Work out the finished part from the listing and answer in its coordinate system (mm). Face numbers are marked on the shaded views. Round coordinates to 2 decimals unless told otherwise and drop trailing zeros. Order: outer loops, then holes, each group sorted by start corner. A loop starts at its lowest first (then second) coordinate and runs counter-clockwise, first axis right, second up. Notation, with made-up numbers: (-32, 8) -> (-4, 8) arc R29 ccw to (-4, 42) -> close; hole circle Ø11 at (-13, -29). An arc over 180 degrees is marked (long way). Use one line per item in the form item = value.
Autodesk Inventor part; units mm, degrees
ref_plane "YZ Plane" through (0, 0, 0) normal (1, 0, 0) x (0, 1, 0)
ref_plane "XZ Plane" through (0, 0, 0) normal (0, 1, 0) x (-1, 0, 0)
ref_plane "XY Plane" through (0, 0, 0) normal (0, 0, 1) x (1, 0, 0)
sketch "Sketch1" plane through (0, 0, 0) normal (0, 1, 0) x (-1, 0, 0)
  circle A0 centre (0, 0) radius 3.2
  circle A1 centre (0, 0) radius 6.5
  line L0 (-2.7713, 1.6) -> (2.7713, 1.6)
  dimension "d0" = 6.4
  dimension "d2" = 13
  dimension "d7" = 4.8
extrude "Extrusion1" add sketch "Sketch1" along normal blind 11 contours A0 L0 | L0 A0 | A1
extrude "Extrusion2" cut sketch "Sketch1" along normal blind 2.7 contours A0 L0 | L0 A0
extrude "Extrusion3" cut sketch "Sketch1" along normal blind 9.7 contours A0 L0 picked at (-0.1715, -0.3975)
sketch "Sketch3" plane through (0, 0, 0) normal (1, 0, 0) x (0, 1, 0)
  line L0 (0, 6.5) -> (11, 6.5)
  line L1 (11, 6.5) -> (11, -6.5)
  line L2 (11, -6.5) -> (0, -6.5)
  line L3 (0, -6.5) -> (0, -3.2)
  line L4 (0, -3.2) -> (9.7, -3.2)
  line L5 (9.7, -3.2) -> (9.7, 1.6)
  line L6 (9.7, 1.6) -> (2.7, 1.6)
  line L7 (2.7, 1.6) -> (2.7, 3.2)
  line L8 (2.7, 3.2) -> (0, 3.2)
  line L9 (0, 3.2) -> (0, 6.5)
  line L10 (11, 1.9375) -> (7, 6.5)
  point P0 (0, 0)
  dimension "d12" = 1.2
  dimension "d13" = 7
extrude "Extrusion5" cut sketch "Sketch3" along normal through all both and the other way through all contours L0 L1 L10
equation "\"offset\" = 0.2"
properties part number "knob"
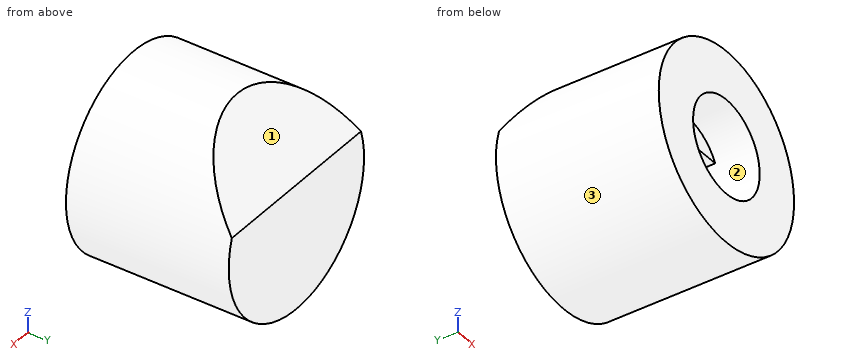
Item 1: The part is cut by section A-A, the plane x = 0. Give the vertices of the cut face in (y, z), and give its area (3 significant figures).
Findings:
outline = (0, -6.5) -> (11, -6.5) -> (11, 1.94) -> (7, 6.5) -> (0, 6.5) -> (0, 3.2) -> (2.7, 3.2) -> (2.7, 1.6) -> (9.7, 1.6) -> (9.7, -3.2) -> (0, -3.2) -> close
area = 83.0 mm^2
Item 2: Consider line 1 along Z through (x, y) = (0, 5.5); line 2 along X through (y, z) = (4.5, 0); line 3 along Z through (x, y) = (-1.5, 3.75). Determine where each line is inside the solid, lowest interval first.
Findings:
line_1 = -6.5 to -3.2, 1.6 to 6.5
line_2 = -6.5 to -3.2, 3.2 to 6.5
line_3 = -6.32 to -2.83, 1.6 to 6.32
Item 3: The part is cut by section D-D, the plane x = 2.5. Give the vertices of the cut face in (y, z), and give its area (3 significant figures).
Findings:
outline = (0, -6) -> (11, -6) -> (11, 1.94) -> (7.44, 6) -> (0, 6) -> (0, 2) -> (2.7, 2) -> (2.7, 1.6) -> (9.7, 1.6) -> (9.7, -2) -> (0, -2) -> close
area = 88.8 mm^2
Item 4: Determine the mould class of the marked faces 1, 2 and 3 for opening direction X: released by +X, released by -X, zero draft, split by the parting line, or undercut.
Findings:
face_1 = zero draft
face_2 = undercut
face_3 = split by the parting line
Item 5: The part is cut by section C-C, the plane z = -0.5. Give the vertices of the cut face in (x, y), and give its area (3 significant figures).
Findings:
outline = (-6.48, 0) -> (-3.16, 0) -> (-3.16, 9.7) -> (3.16, 9.7) -> (3.16, 0) -> (6.48, 0) -> (6.48, 11) -> (-6.48, 11) -> close
area = 81.3 mm^2
Item 6: Flat-ended cylindrical pins translate along their axes: P1, Ø2, axis at x = 3.5, y = 2, coming from the +Z side; P2, Ø1.3, axis at x = 1, z = 2, coming from the -Y side; P3, Ø1.4, axis at x = -1, z = 0, coming from the -Y side. Find the tip coordinate at first contact, or state that the pin passes through.
Findings:
P1 = 6
P2 = 2.7
P3 = 9.7
Item 7: The part is cut by section B-B, the plane y = 5. Give the vertices of the cut face in (x, z).
Findings:
outline = circle Ø13 at (0, 0); hole (-2.77, 1.6) arc R3.2 ccw (long way) to (2.77, 1.6) -> close
